Autodesk Fusion 360 part; units mm, degrees
sketch "main" plane through (0, 0, 0) normal (0, 0, 1) x (1, 0, 0) in component "crank-arm"
  circle A0 centre (0, 0) radius 13.05
  circle A1 centre (0, 0) radius 23
  line L0 (-23, 0) -> (23, 0)
  line L1 (23, 0) -> (23, -120)
  line L2 (23, -120) -> (-23, -120)
  line L3 (-23, -120) -> (-23, 0)
  circle A2 centre (0, -120) radius 23
  circle A3 centre (0, -120) radius 13.05
  dimension "d1" = 26.1
  dimension "d2" = 46
  dimension "d3" = 46
  dimension "d4" = 120
  dimension "d5" = 46
  dimension "d6" = 26.1
extrude "Extrude1" add sketch "main" along normal blind 8 contours A0 L0 | A0 A1 L0 | A0 A1 L0 | A0 L0 | A1 L1 L3 A2 | L2 A2 A3 | L2 A2 A3 in component "crank-arm"
extrude "Extrude2" add sketch "main" along normal blind 7.5 from surface at 8 contours A0 A1 L0 | A0 A1 L0 | A1 L1 L3 A2 | L2 A2 A3 | L2 A2 A3 | L2 A3 | L2 A3 in component "crank-arm"
chamfer "Chamfer1" distance 2.5 angle 45 8 edges at (-23, -60, 15.5) (0, -143, 15.5) (23, -60, 15.5) (0, 23, 15.5) (-23, -60, 0) (0, 23, 0) (23, -60, 0) (0, -143, 0) in component "crank-arm"
component "crank-arm" placed x (1, 0, 0) y (0, 1, 0) z (0, 0, 1) at (0, 0, 0)
equation "d1 = 26 mm + 0.1 mm"
equation "d6 = 26 mm + 0.1 mm"
equation "d10 = 8 mm - 0.5 mm"
For this review, take the finished solid that the model builds, in its own axes (mm). A direction names the side the tool comes from. Give positions to 0.01 mm unless a question says otherwise; leave off trailing zeros. Write each loop counter-clockwise with the first axis right and the second up, starting at its lowest first coordinate (ties: lowest second). Pieces come first, ordered by that corner, then holes.
Item 1: Take a section at A-A (x = 0). Give the boundary of the cut face in (y, z), and give its area (3 significant figures).
Item 2: Machinability: for faces 4 (the face through (-9.62, -8.82, 11.7)), 5 (the face through (-1.7, -132.94, 3.94)), 6 (the face through (0.454, 20.651, 0.156)), which of the approach directions +Z, -Z, +X, -X, +Y, -Y give a long, thin tool a straight path to every point of the face, cutting with its end or side? Answer none if there is none.
Item 3: The part is to be moulded in two halves that separate along Y. For faces 1 (the face through (23, -59, 8)), 2 (the face through (0, 21, 15)), 3 (the face through (0, 0, 8)), say which applies: +Y half, -Y half, draft (parallel to the pull), parting line (faces both ways), or undercut.
Item 4: Take a section at D-D (y = -6.5). Give the boundary of the cut face in (x, z), and give its area (3 significant figures).
Item 5: Insertion check: P1, Ø1.5, axis at x = 16.5, z = 1.5, coming from the +Y side; P2, Ø4, axis at x = 16.5, z = 9, coming from the -Y side; P3, Ø4, axis at x = -2.5, z = 8.5, coming from the +Y side. Each pin has a flat end and moves straight along its axis. Give the tip position at first contact, or say it passes through.
Item 6: Wall thickness on probe 1 along X at (y, z) = (0, 9.5); probe 2 along Y at (x, z) = (0, 12); probe 3 along Y at (x, z) = (0, 3.75): over which ranges is each line inside the solid? List them lowest first.
Item 7: Take a section at B-B (z = 11). Give the boundary of the cut face in (x, y).
Item 8: Take a section at C-C (y = -89). Give the boundary of the cut face in (x, z), and give its area (4 significant figures).
Established:
1. outline: (-143, 2.5) - (-140.5, 0) - (-133.05, 0) - (-133.05, 8) - (-106.95, 8) - (-106.95, 0) - (20.5, 0) - (23, 2.5) - (23, 13) - (20.5, 15.5) - (13.05, 15.5) - (13.05, 8) - (-13.05, 8) - (-13.05, 15.5) - (-140.5, 15.5) - (-143, 13) - close
1. area: 2,160 mm2
2. face 4: +Z
2. face 5: -Z
2. face 6: -Z, +Y
3. face 1: draft
3. face 2: +Y half
3. face 3: undercut
4. outline: (-23, 2.5) - (-20.5, 0) - (20.5, 0) - (23, 2.5) - (23, 13) - (20.5, 15.5) - (11.32, 15.5) - (11.32, 8) - (-11.32, 8) - (-11.32, 15.5) - (-20.5, 15.5) - (-23, 13) - close
4. area: 531 mm2
5. P1: stops at y = 15.91
5. P2: stops at y = -137.85
5. P3: stops at y = 22.99
6. probe 1: x = -23 to -13.05, 13.05 to 23
6. probe 2: y = -143 to -13.05, 13.05 to 23
6. probe 3: y = -143 to -133.05, -106.95 to 23
7. outline: (-23, -120) arc R23 ccw to (23, -120) - (23, 0) arc R23 ccw to (-23, 0) - close; hole circle Ø26.1 at (0, 0)
8. outline: (-23, 2.5) - (-20.5, 0) - (20.5, 0) - (23, 2.5) - (23, 13) - (20.5, 15.5) - (-20.5, 15.5) - (-23, 13) - close
8. area: 700.5 mm2
